Study the drawing (mm; zero at the part's minimum x, y, z) and answer. Round coordinates to 2 decimals unless told otherwise and drop trailing zeros. Write each loop counter-clockwise with the first axis right and the second up, starting at its lowest first coordinate (ties: lowest second). Pieces come first, ordered by that corner, then holes.
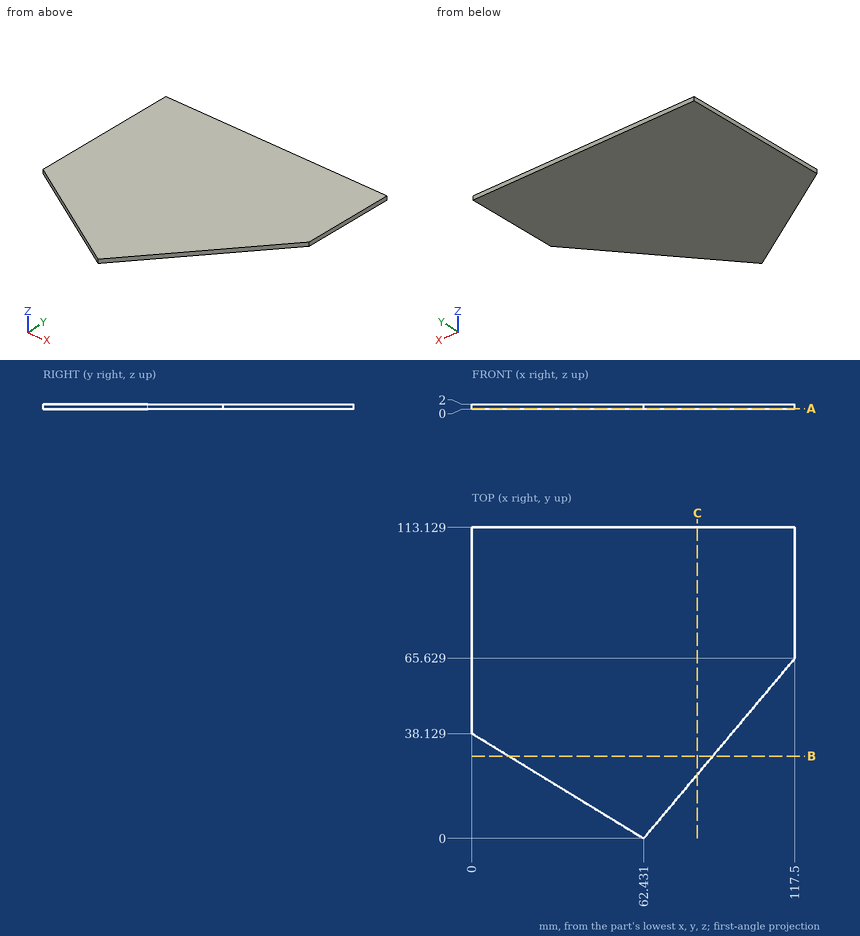
1. Section B-B on y = 30 is taken. Determine the outline of the cut face in (x, z).
Geometry says:
outline: (13.31, 0) - (87.6, 0) - (87.6, 2) - (13.31, 2) - close
2. Section C-C on x = 82 is taken. Determine the outline of the cut face in (y, z), plus the area to 3 significant figures.
Geometry says:
outline: (23.32, 0) - (113.13, 0) - (113.13, 2) - (23.32, 2) - close
area: 180 mm2
3. Given pin 1 (6 mm diameter, centred on x = 50.5, y = 28.5, fed in from -Z), flat-ended and moving along its own axis, determine where the tip first touches the part or whether it passes through.
Geometry says:
pin 1: stops at z = 0
4. Straight lines are drawn through the part: line 1 along X through (y, z) = (29.5, 0.85) (1 decimal); line 2 along Y through (x, z) = (90.5, 0.7); line 3 along Y through (x, z) = (76, 1.15). For each, find the intervals that lie inside material, in ascending order.
Geometry says:
line 1: x = 14.1 to 87.2
line 2: y = 33.45 to 113.13
line 3: y = 16.17 to 113.13
5. Section A-A on z = 0.3 is taken. Determine the outline of the cut face in (x, y), plus the area to 3 significant figures.
Geometry says:
outline: (0, 38.13) - (62.43, 0) - (117.5, 65.63) - (117.5, 113.13) - (0, 113.13) - close
area: 10,300 mm2
